from build123d import *

# Parameters (mm, degrees)
SKETCH1_W           = 85
SKETCH1_H           = 70
BOSS_EXTRUDE1_DEPTH = 5
BOSS_EXTRUDE2_DEPTH = 7.5
FILLET1_R           = 1.5
FILLET2_R           = 20


with BuildPart() as part:
    # Sketch1 → Boss-Extrude1 (new body)
    with BuildSketch(Plane(origin=(0, 0, 0), x_dir=(1, 0, 0), z_dir=(0, 1, 0))):
        with Locations((42.5, -35)):
            Rectangle(SKETCH1_W, SKETCH1_H)
    extrude(amount=BOSS_EXTRUDE1_DEPTH)

    # Sketch2 → Boss-Extrude2 (add)
    with BuildSketch(Plane(origin=(0, 5, 0), x_dir=(1, 0, 0), z_dir=(0, 1, 0))):
        with BuildLine():
            ThreePointArc((31.712705589, -32.714866344), (24.490905169, -31.43108309), (30.560453247, -35.549709909))
            Line((30.560453247, -35.549709909), (27.964899606, -32.843125107))
            Line((27.964899606, -32.843125107), (31.712705589, -32.714866344))
        make_face()
        with BuildLine():
            Line((27.964899606, -32.843125107), (30.560453247, -35.549709909))
            ThreePointArc((30.560453247, -35.549709909), (31.41423477, -34.314378627), (31.714899606, -32.843125107))
            ThreePointArc((31.714899606, -32.843125107), (31.714351061, -32.778986344), (31.712705589, -32.714866344))
            Line((31.712705589, -32.714866344), (27.964899606, -32.843125107))
        make_face()
        with BuildLine():
            ThreePointArc((52.217093622, -32.013157813), (52.595566686, -33.531135874), (53.560453247, -34.762595649))
            Line((53.560453247, -34.762595649), (55.964899606, -31.884899051))
            Line((55.964899606, -31.884899051), (52.217093622, -32.013157813))
        make_face()
        with BuildLine():
            Line((55.964899606, -31.884899051), (53.560453247, -34.762595649))
            ThreePointArc((53.560453247, -34.762595649), (57.553267661, -35.281895801), (59.714899606, -31.884899051))
            ThreePointArc((59.714899606, -31.884899051), (55.900760842, -28.135447595), (52.217093622, -32.013157813))
            Line((52.217093622, -32.013157813), (55.964899606, -31.884899051))
        make_face()
        with BuildLine():
            Line((42.5, -48), (42.5, -51.75))
            ThreePointArc((42.5, -51.75), (45.151650429, -50.651650429), (46.25, -48))
            ThreePointArc((46.25, -48), (45.89699675, -46.411631945), (44.904446358, -45.122303402))
            Line((44.904446358, -45.122303402), (42.5, -48))
        make_face()
        with BuildLine():
            ThreePointArc((39.904446358, -45.293415198), (39.020618373, -49.398714944), (42.5, -51.75))
            Line((42.5, -51.75), (42.5, -48))
            Line((42.5, -48), (39.904446358, -45.293415198))
        make_face()
        with BuildLine():
            Line((39.904446358, -45.293415198), (42.5, -48))
            Line((42.5, -48), (44.904446358, -45.122303402))
            ThreePointArc((44.904446358, -45.122303402), (42.371741238, -44.252194017), (39.904446358, -45.293415198))
        make_face()
    extrude(amount=BOSS_EXTRUDE2_DEPTH)

    # Fillet1
    fillet1_edges = [part.edges().sort_by_distance(p)[0] for p in [
        (25.369345964, 12.5, 30.136540305),
        (59.712705589, 12.5, 31.756640288),
        (45.095553642, 12.5, 50.706584802),
    ]]
    fillet(fillet1_edges, radius=FILLET1_R)

    # Fillet2
    fillet2_edges = [part.edges().sort_by_distance(p)[0] for p in [
        (0, 2.5, 0),
        (85, 2.5, 0),
        (85, 2.5, 70),
        (0, 2.5, 70),
    ]]
    fillet(fillet2_edges, radius=FILLET2_R)


solid = part.part
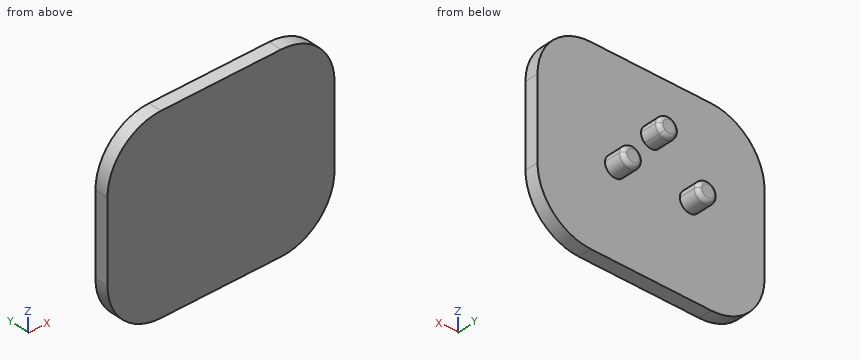
The listing builds one solid part. Answer for the finished solid, in the listing's coordinates (mm). Give positions to 0.01 mm unless a question says otherwise; leave off trailing zeros. Order: outer loops, then holes, each group sorted by start corner. A loop starts at its lowest first (then second) coordinate and runs counter-clockwise, first axis right, second up. Notation, with made-up numbers: (86, -6) - (104, -6) arc R17 cw to (104, 10) - close; hole circle Ø11 at (22.25, 11). An arc over 180 degrees is marked (long way). Use one line per item in the form item = value.
1) Find section C-C on z = 25. Determine the outline of the cut face in (x, y), and give its area (3 significant figures).
Verdict:
outline = (0, 0) - (85, 0) - (85, 5) - (0, 5) - close
area = 425 mm^2
2) Each of these flat-tipped pins is pushed along its axis until it touches: pin 1 (1 mm diameter, centred on x = 50.5, z = 28, fed in from +Y); pin 2 (1.5 mm diameter, centred on x = 24.5, y = 8.5, fed in from +Z). Where does it stop, or does it pass through?
Verdict:
pin_1 = 5
pin_2 = 35.43
3) Find section A-A on y = 6.5. Determine the outline of the cut face in (x, z), and give its area (3 significant figures).
Verdict:
outline = (31.71, 32.71) arc R3.75 ccw to (31.71, 32.84) arc R3.75 ccw (long way) to start; circle Ø7.5 at (42.5, 48); circle Ø7.5 at (55.96, 31.88)
area = 133 mm^2
4) Consider probe 1 along Y at (x, z) = (22, 28); probe 2 along X at (y, z) = (11.25, 33); probe 3 along Z at (x, y) = (5, 2.75). Determine where each line is inside the solid, lowest interval first. Write a range as [from, to].
Verdict:
probe_1 = [0, 5]
probe_2 = [24.24, 31.69], [52.41, 59.52]
probe_3 = [6.77, 63.23]
5) Find section B-B on x = 47.5. Determine the outline of the cut face in (y, z), and give its area (3 significant figures).
Verdict:
outline = (0, 0) - (5, 0) - (5, 70) - (0, 70) - close
area = 350 mm^2
